Could you check a few things on this model? Use its own coordinates, in mm. A direction names the side the tool comes from. Coordinates: 2 decimals unless noted, no trailing zeros. Write each loop counter-clockwise with the first axis right and the second up, starting at its lowest first coordinate (ties: lowest second). Pieces come first, ordered by that corner, then holes.
```python
from build123d import *

# Parameters (mm, degrees)
SKETCH_1_W          = 15
SKETCH_1_H          = 6
SKETCH_1_W_2        = 13
SKETCH_1_H_2        = 4
EXTRUDE_1_DEPTH     = 400
SKETCH_2_R          = 1.5
CUT_EXTRUDE_1_DEPTH = 10
SKETCH_3_R          = 1.6
SKETCH_3_R_2        = 1.5
CUT_EXTRUDE_2_DEPTH = 401.115295884
SKETCH_4_W          = 23.248970848
SKETCH_4_H          = 9.936482471
CUT_EXTRUDE_3_DEPTH = 10


with BuildPart() as part:
    # 草图1 → 凸台-拉伸1 (new body)
    with BuildSketch(Plane.XY):
        Rectangle(SKETCH_1_W, SKETCH_1_H)
        Rectangle(SKETCH_1_W_2, SKETCH_1_H_2, mode=Mode.SUBTRACT)
    extrude(amount=EXTRUDE_1_DEPTH)

    # 草图2 → 切除-拉伸1 (cut)
    with BuildSketch(Plane.XZ.offset(3)):
        with Locations(Location((3.5, 35, 0), (0, 0, 270))):
            Circle(SKETCH_2_R)
        with Locations(Location((3.5, 9, 0), (0, 0, 270))):
            Circle(SKETCH_2_R)
        with Locations(Location((-3.5, 22, 0), (0, 0, 270))):
            Circle(SKETCH_2_R)
        with Locations(Location((0, 48, 0), (0, 0, 270))):
            Circle(SKETCH_2_R)
    extrude(amount=-CUT_EXTRUDE_1_DEPTH, mode=Mode.SUBTRACT)

    # 草图3 → 切除-拉伸2 (cut, through all)
    with BuildSketch(Plane(origin=(0, 3, 0), x_dir=(1, 0, 0), z_dir=(0, 1, 0))):
        with Locations(Location((0, -335, 0), (0, 0, 270))):
            Circle(SKETCH_3_R)
        with Locations(Location((0, -327, 0), (0, 0, 270))):
            Circle(SKETCH_3_R)
        with Locations(Location((0, -198.5, 0), (0, 0, 270))):
            Circle(SKETCH_3_R)
        with Locations(Location((0, -276, 0), (0, 0, 270))):
            Circle(SKETCH_3_R)
        with Locations(Location((0, -268, 0), (0, 0, 270))):
            Circle(SKETCH_3_R)
        with Locations(Location((4, -396, 0), (0, 0, 270))):
            Circle(SKETCH_3_R_2)
        with Locations(Location((-4, -396, 0), (0, 0, 90))):
            Circle(SKETCH_3_R_2)
        with Locations(Location((0, -221, 0), (0, 0, 270))):
            Circle(SKETCH_3_R)
        with Locations(Location((0, -213, 0), (0, 0, 270))):
            Circle(SKETCH_3_R)
        with Locations(Location((0, -158.5, 0), (0, 0, 270))):
            Circle(SKETCH_3_R)
        with Locations(Location((0, -143.5, 0), (0, 0, 270))):
            Circle(SKETCH_3_R)
        with Locations(Location((0, -120.5, 0), (0, 0, 270))):
            Circle(SKETCH_3_R)
        with Locations(Location((0, -128.5, 0), (0, 0, 270))):
            Circle(SKETCH_3_R)
        with Locations(Location((0, -75.5, 0), (0, 0, 270))):
            Circle(SKETCH_3_R)
        with Locations(Location((0, -83.5, 0), (0, 0, 270))):
            Circle(SKETCH_3_R)
        with Locations(Location((0, -380, 0), (0, 0, 270))):
            Circle(SKETCH_3_R)
        with Locations(Location((0, -322, 0), (0, 0, 270))):
            Circle(SKETCH_3_R)
    extrude(amount=-CUT_EXTRUDE_2_DEPTH, mode=Mode.SUBTRACT)

    # 草图4 → 切除-拉伸3 (cut)
    with BuildSketch(Plane(origin=(0, 3, 0), x_dir=(1, 0, 0), z_dir=(0, 1, 0))):
        with Locations((0, -0.031758764)):
            Rectangle(SKETCH_4_W, SKETCH_4_H)
    extrude(amount=-CUT_EXTRUDE_3_DEPTH, mode=Mode.SUBTRACT)


solid = part.part
```
1. Please list where these lines run through material, in increasing order: line 1 along Y through (x, z) = (5.5, 198.5); line 2 along X through (y, z) = (2.3, 322); line 3 along X through (y, z) = (1.2, 233).
Verdict:
line 1: y = -3 to -2, 2 to 3
line 2: x = -7.5 to -1.6, 1.6 to 7.5
line 3: x = -7.5 to -6.5, 6.5 to 7.5
2. I want a section at B-B on y = -1. Please give me the cut outline in (x, z).
Verdict:
outline: (-7.5, 5) - (-6.5, 5) - (-6.5, 400) - (-7.5, 400) - close; (6.5, 5) - (7.5, 5) - (7.5, 400) - (6.5, 400) - close
3. If we mould it in two halves opening along X, with no side actions, what happens to faces 1 (the face through (-2, -3, 200)), 2 (the face through (7.5, 0, 200)), 3 (the face through (-2, 2, 200))? For each: pulls with the +X half, pulls with the -X half, needs draft (parallel to the pull), parting line crosses it, or undercut.
Verdict:
face 1: needs draft
face 2: pulls with the +X half
face 3: undercut
4. On a 3-axis mill with a long thin cutter (end or side, diameter ignored), from which of +Z, -Z, +X, -X, +Y, -Y can I reach the whole of each face in a straight line? I mean faces 4 (the face through (-2, -2, 200)), 5 (the face through (-2, 3, 200)). Say none if no direction works.
Verdict:
face 4: +Z, -Z
face 5: +Z, -Z, +X, -X, +Y
5. I want a section at A-A on z = 70. Please give me the cut outline in (x, y), plus the area to 3 significant figures.
Verdict:
outline: (-7.5, -3) - (7.5, -3) - (7.5, 3) - (-7.5, 3) - close; hole (-6.5, -2) - (6.5, -2) - (6.5, 2) - (-6.5, 2) - close
area: 38.0 mm2
